Can you work these out from the model? Positions are in its coordinate system, mm. Face numbers are marked on the shaded views. A direction names the side the tool comes from. Coordinates: 2 decimals unless noted, no trailing zeros. Write each loop counter-clockwise with the first axis right and the second up, starting at its lowest first coordinate (ties: lowest second). Pieces come first, ordered by that corner, then holes.
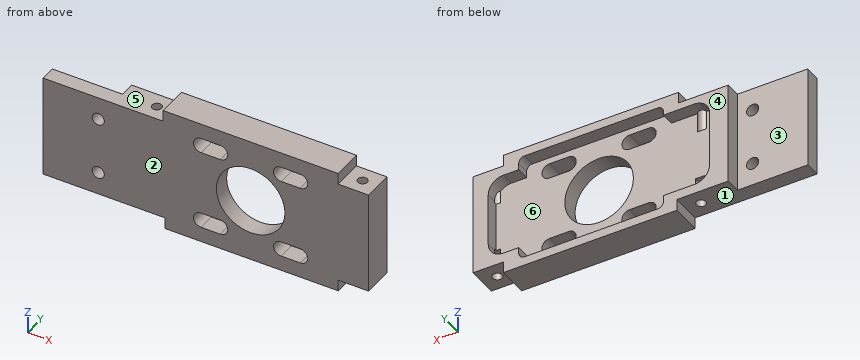
```python
from build123d import *

# Parameters (mm, degrees)
EXTRUDE_1_DEPTH      = 8
SKETCH_2_W           = 18.5
SKETCH_2_H           = 27
CUT_EXTRUDE_1_DEPTH  = 4
SKETCH_3_R           = 1.6
CUT_EXTRUDE_2_DEPTH  = 5
SKETCH_4_R           = 9
CUT_EXTRUDE_3_DEPTH  = 9
CUT_EXTRUDE_4_DEPTH  = 3.5
SKETCH_6_R           = 1.25
CUT_EXTRUDE_8_DEPTH  = 7
SKETCH_7_R           = 1.25
CUT_EXTRUDE_9_DEPTH  = 7
SKETCH_8_R           = 1.25
CUT_EXTRUDE_10_DEPTH = 7
SKETCH_9_R           = 1.25
CUT_EXTRUDE_11_DEPTH = 7


with BuildPart() as part:
    # Эскиз1 → Бобышка-Вытянуть1 (new body)
    with BuildSketch(Plane(origin=(0, 0, 0), x_dir=(1, 0, 0), z_dir=(0, 1, 0))):
        Polygon((43, 13.5), (43, -13.5), (35, -13.5), (35, -16.5), (-11, -16.5), (-11, -13.5), (-42.5, -13.5), (-42.5, 13.5), (-10.5, 13.5), (-10.5, 16.5), (35, 16.5), (35, 13.5), align=None)
    extrude(amount=EXTRUDE_1_DEPTH)

    # Эскиз2 → Вырез-Вытянуть1 (cut)
    with BuildSketch(Plane(origin=(0, 8, 0), x_dir=(1, 0, 0), z_dir=(0, 1, 0))):
        with Locations((-33.25, 0)):
            Rectangle(SKETCH_2_W, SKETCH_2_H)
    extrude(amount=-CUT_EXTRUDE_1_DEPTH, mode=Mode.SUBTRACT)

    # Эскиз3 → Вырез-Вытянуть2 (cut, through all)
    with BuildSketch(Plane(origin=(0, 4, 0), x_dir=(1, 0, 0), z_dir=(0, 1, 0))):
        with Locations(Location((-28, 7.5, 0), (0, 0, 270))):  # turned: the seam where the file's is
            Circle(SKETCH_3_R)
        with Locations(Location((-28, -7.5, 0), (0, 0, 90))):  # turned: the seam where the file's is
            Circle(SKETCH_3_R)
    extrude(amount=-CUT_EXTRUDE_2_DEPTH, mode=Mode.SUBTRACT)

    # Эскиз4 → Вырез-Вытянуть3 (cut, through all)
    with BuildSketch(Plane.XZ):
        with Locations(Location((12, 0, 0), (0, 0, 270))):  # turned: the seam where the file's is
            Circle(SKETCH_4_R)
        with BuildLine():
            Line((20, 12.5), (25, 12.5))
            ThreePointArc((25, 12.5), (27, 10.5), (25, 8.5))
            Line((25, 8.5), (20, 8.5))
            ThreePointArc((20, 8.5), (18, 10.5), (20, 12.5))
        make_face()
        with BuildLine():
            Line((4, 12.5), (-1, 12.5))
            ThreePointArc((-1, 12.5), (-3, 10.5), (-1, 8.5))
            Line((-1, 8.5), (4, 8.5))
            ThreePointArc((4, 8.5), (6, 10.5), (4, 12.5))
        make_face()
        with BuildLine():
            Line((20, -12.5), (25, -12.5))
            ThreePointArc((25, -12.5), (27, -10.5), (25, -8.5))
            Line((25, -8.5), (20, -8.5))
            ThreePointArc((20, -8.5), (18, -10.5), (20, -12.5))
        make_face()
        with BuildLine():
            Line((4, -12.5), (-1, -12.5))
            ThreePointArc((-1, -12.5), (-3, -10.5), (-1, -8.5))
            Line((-1, -8.5), (4, -8.5))
            ThreePointArc((4, -8.5), (6, -10.5), (4, -12.5))
        make_face()
    extrude(amount=-CUT_EXTRUDE_3_DEPTH, mode=Mode.SUBTRACT)

    # Эскиз5 → Вырез-Вытянуть4 (cut)
    with BuildSketch(Plane(origin=(0, 8, 0), x_dir=(1, 0, 0), z_dir=(0, 1, 0))):
        with BuildLine():
            Line((-19.099474061, 7.023433075), (-19.099474061, -7.604302917))
            ThreePointArc((-19.099474061, -7.604302917), (-17.927901185, -10.432730042), (-15.099474061, -11.604302917))
            Line((-15.099474061, -11.604302917), (-7, -11.604302917))
            Line((-7, -11.604302917), (-7, -12.7))
            ThreePointArc((-7, -12.7), (-6.560660172, -13.760660172), (-5.5, -14.2))
            Line((-5.5, -14.2), (29.5, -14.2))
            ThreePointArc((29.5, -14.2), (30.560660172, -13.760660172), (31, -12.7))
            Line((31, -12.7), (31, -10.901181177))
            Line((31, -10.901181177), (35, -10.901181177))
            ThreePointArc((35, -10.901181177), (37.828427125, -9.729608302), (39, -6.901181177))
            Line((39, -6.901181177), (39, 7.023433075))
            ThreePointArc((39, 7.023433075), (37.828427125, 9.8518602), (35, 11.023433075))
            Line((35, 11.023433075), (31, 11.023433075))
            Line((31, 11.023433075), (31, 12.7))
            ThreePointArc((31, 12.7), (30.560660172, 13.760660172), (29.5, 14.2))
            Line((29.5, 14.2), (-5.5, 14.2))
            ThreePointArc((-5.5, 14.2), (-6.560660172, 13.760660172), (-7, 12.7))
            Line((-7, 12.7), (-7, 11.023433075))
            Line((-7, 11.023433075), (-15.099474061, 11.023433075))
            ThreePointArc((-15.099474061, 11.023433075), (-17.927901185, 9.8518602), (-19.099474061, 7.023433075))
        make_face()
    extrude(amount=-CUT_EXTRUDE_4_DEPTH, mode=Mode.SUBTRACT)

    # Эскиз6 → Вырез-Вытянуть8 (cut)
    with BuildSketch(Plane.XY.offset(13.5)):
        with Locations((39, 4)):
            Circle(SKETCH_6_R)
    extrude(amount=-CUT_EXTRUDE_8_DEPTH, mode=Mode.SUBTRACT)

    # Эскиз7 → Вырез-Вытянуть9 (cut)
    with BuildSketch(Plane.XY.offset(13.5)):
        with Locations((-15, 4)):
            Circle(SKETCH_7_R)
    extrude(amount=-CUT_EXTRUDE_9_DEPTH, mode=Mode.SUBTRACT)

    # Эскиз8 → Вырез-Вытянуть10 (cut)
    with BuildSketch(Plane(origin=(0, 0, -13.5), x_dir=(-1, 0, 0), z_dir=(0, 0, -1))):
        with Locations(Location((-39, 4, 0), (0, 0, 180))):  # turned: the seam where the file's is
            Circle(SKETCH_8_R)
    extrude(amount=-CUT_EXTRUDE_10_DEPTH, mode=Mode.SUBTRACT)

    # Эскиз9 → Вырез-Вытянуть11 (cut)
    with BuildSketch(Plane(origin=(0, 0, -13.5), x_dir=(-1, 0, 0), z_dir=(0, 0, -1))):
        with Locations((14.5, 4)):
            Circle(SKETCH_9_R)
    extrude(amount=-CUT_EXTRUDE_11_DEPTH, mode=Mode.SUBTRACT)


solid = part.part
```
1. Which directions (+Z, -Z, +X, -X, +Y, -Y) give clear straight access to the entire face, cutting with the end or side of a thin tool? Please do the marked faces 1, 2 and 3.
2. We'd pull the mould along Z, two halves only. Please class the marked faces 4, 5 and 6: released by +Z, released by -Z, zero draft, split by the parting line, or undercut.
3. If we section it at C-C, the plane z = -2.5: List the corners of the cut face in (x, y) for me.
4. I'm going to push flat-ended pins straight in: P1, Ø6, axis at x = 27, z = 9, coming from the +Y side; P2, Ø2.5, axis at x = 41, y = 5.5, coming from the -Z side; P3, Ø2.5, axis at y = 3, z = -15, coming from the +X side. Where does each tip first touch, or does it pass through?
5. If we section it at D-D, the plane x = 14.5: List the corners of the cut face in (y, z) for me, plus the area to 3 significant figures.
6. If we section it at B-B, the plane x = -28: List the corners of the cut face in (y, z) for me, plus the area to 3 significant figures.
7. If I drill on L1, parallel to X at y = 0.5, z = -10; L2, parallel to Z at x = 26, y = 7; L3, parallel to X at y = 3.65, z = 0, over which ranges is the centre line in solid material (lowest first)?
Answers:
1. face 1: -Z, -X, +Y, -Y
1. face 2: +Z, -Z, +X, -X, -Y
1. face 3: +Z, -Z, -X, +Y
2. face 4: zero draft
2. face 5: released by +Z
2. face 6: undercut
3. outline: (-42.5, 0) - (3.35, 0) - (3.35, 4.5) - (-19.1, 4.5) - (-19.1, 8) - (-24, 8) - (-24, 4) - (-42.5, 4) - close; (20.65, 0) - (43, 0) - (43, 8) - (39, 8) - (39, 4.5) - (20.65, 4.5) - close
4. P1: stops at y = 4.5
4. P2: stops at z = -13.5
4. P3: stops at x = 35
5. outline: (0, -16.5) - (8, -16.5) - (8, -14.2) - (4.5, -14.2) - (4.5, -8.65) - (0, -8.65) - close; (0, 8.65) - (4.5, 8.65) - (4.5, 14.2) - (8, 14.2) - (8, 16.5) - (0, 16.5) - close
5. area: 86.8 mm2
6. outline: (0, -13.5) - (4, -13.5) - (4, -9.1) - (0, -9.1) - close; (0, -5.9) - (4, -5.9) - (4, 5.9) - (0, 5.9) - close; (0, 9.1) - (4, 9.1) - (4, 13.5) - (0, 13.5) - close
6. area: 82.4 mm2
7. L1: x = -42.5 to -2.94, 5.94 to 18.06, 26.94 to 43
7. L2: z = -16.5 to -14.2, 14.2 to 16.5
7. L3: x = -42.5 to 3, 21 to 43
